Answer from the drawing. Dimensions are ordinates in mm from the lowest x, y and z of the part. A direction names the side the tool comes from. Coordinates: 2 decimals unless noted, no trailing zeros. Order: outer loops, then holes, each group sorted by start corner. A loop starts at its lowest first (then second) coordinate and runs counter-clockwise, first axis right, second up. Notation, with made-up numbers: (69.5, 26) - (97.5, 26) arc R36 cw to (97.5, 63) - close; hole circle Ø9 at (83.25, -27.5). An arc over 180 degrees is marked (long way). Use a Markdown table: item, result. Add a question column.
Item 1: Flat-ended cylindrical pins translate along their axes: P1, Ø6, axis at y = 68.5, z = 53.5, coming from the +X side; P2, Ø1, axis at y = 86, z = 10.5, coming from the +X side (1 decimal). Find the tip coordinate at first contact, or state that the pin passes through.
Item 2: For the marked faces 1 and 2, determine the directions among +Z, -Z, +X, -X, +Y, -Y from which every point of the face is accessible in a straight line to the end or side of a thin tool.
Item 3: The part is cut by section B-B, the plane z = 47. Give the vertices of the cut face in (x, y), then the cut area to 3 significant figures.
Item 4: The part is cut by section C-C, the plane x = 39. Give the vertices of the cut face in (y, z), then the cut area to 3 significant figures.
Item 5: The part is cut by section D-D, the plane x = 113.5. Give the vertices of the cut face in (y, z) (1 decimal).
Item 6: Find the intervals of material crossed by line 1 along Z through (x, y) = (106, 50.5) (1 decimal); line 2 along Y through (x, z) = (54, 28); line 3 along X through (y, z) = (91.5, 20) (1 decimal), in increasing order.
Item 7: The mould has two halves that part along X. Classify the marked faces 3, 4 and 5: released by +X, released by -X, zero draft, split by the parting line, or undercut.
Item 8: The part is cut by section A-A, the plane y = 80.5. Give the vertices of the cut face in (x, z) (1 decimal).
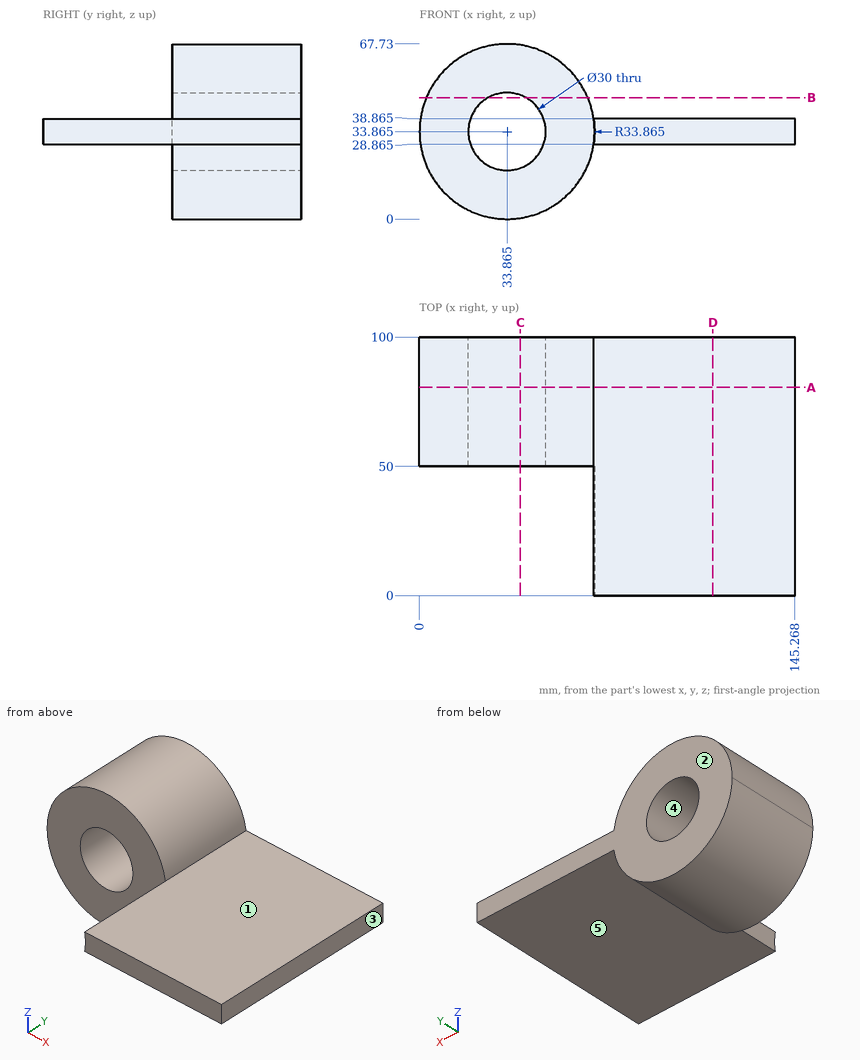
Solution:
| question | item | result |
|---|---|---|
| 1 | P1 | stops at x = 63.36 |
| 1 | P2 | stops at x = 58.8 |
| 2 | face 1 | +Z, +X, +Y, -Y |
| 2 | face 2 | +Z, -Z, +X, -X, +Y |
| 3 | outline | (2.65, 50) - (26.62, 50) - (26.62, 100) - (2.65, 100) - close; (41.11, 50) - (65.08, 50) - (65.08, 100) - (41.11, 100) - close |
| 3 | area | 2,400 mm2 |
| 4 | outline | (50, 0.39) - (100, 0.39) - (100, 19.77) - (50, 19.77) - close; (50, 47.96) - (100, 47.96) - (100, 67.34) - (50, 67.34) - close |
| 4 | area | 1,940 mm2 |
| 5 | outline | (0, 28.9) - (100, 28.9) - (100, 38.9) - (0, 38.9) - close |
| 6 | line 1 | z = 28.9 to 38.9 |
| 6 | line 2 | y = 50 to 100 |
| 6 | line 3 | x = 3 to 28.1, 39.6 to 64.8 |
| 7 | face 3 | released by +X |
| 7 | face 4 | undercut |
| 7 | face 5 | zero draft |
| 8 | outline | (67.4, 28.9) - (145.3, 28.9) - (145.3, 38.9) - (67.4, 38.9) arc R33.9 ccw (long way) to start; hole circle Ø30 at (33.9, 33.9) |
